```python
from build123d import *

# Parameters (mm, degrees)
REVOLVE_THIN1_OUTLINE_R                   = 10
REVOLVE_THIN1_DEPTH                       = 165
REVOLVE_THIN1_START                       = 15
REVOLVE_THIN1_2_OUTLINE_R                 = 12.5
REVOLVE_THIN1_2_OUTLINE_R_2               = 10
REVOLVE_THIN1_2_DEPTH                     = 10
F_5_0MM_DOWEL_HOLE1_D                     = 5
F_5_0MM_DOWEL_HOLE1_DEPTH                 = 10
F_5_0MM_DOWEL_HOLE1_CSINK_D               = 5.05
F_5_0MM_DOWEL_HOLE1_CSINK_ANGLE           = 90
F_5_0MM_DOWEL_HOLE1_TIP                   = 1.502151548
F_5_0MM_DOWEL_HOLE1_ON_FACE_2_D           = 5
F_5_0MM_DOWEL_HOLE1_ON_FACE_2_DEPTH       = 10
F_5_0MM_DOWEL_HOLE1_ON_FACE_2_CSINK_D     = 5.05
F_5_0MM_DOWEL_HOLE1_ON_FACE_2_CSINK_ANGLE = 90
F_5_0MM_DOWEL_HOLE1_ON_FACE_2_TIP         = 1.502151548
CUT_EXTRUDE1_DEPTH                        = 3


# Read off the part's stored shape, not the designer's step: Revolve-Thin1
with BuildPart() as part:
    # Revolve-Thin1 outline → Revolve-Thin1 (new body)
    with BuildSketch(Plane.YZ):
        Circle(REVOLVE_THIN1_OUTLINE_R)
    extrude(amount=REVOLVE_THIN1_DEPTH)

    # Revolve-Thin1 2 outline → Revolve-Thin1 2 (add)
    with BuildSketch(Plane.YZ.offset(REVOLVE_THIN1_START)):
        Circle(REVOLVE_THIN1_2_OUTLINE_R)
        Circle(REVOLVE_THIN1_2_OUTLINE_R_2, mode=Mode.SUBTRACT)
    extrude(amount=REVOLVE_THIN1_2_DEPTH)

    # Ø5.0mm Dowel Hole1
    with Locations(Plane(origin=(0, 0, 0), x_dir=(0, -1, 0), z_dir=(-1, 0, 0))):
        with Locations((0, 0)):
            CounterSinkHole(F_5_0MM_DOWEL_HOLE1_D / 2, F_5_0MM_DOWEL_HOLE1_CSINK_D / 2, depth=F_5_0MM_DOWEL_HOLE1_DEPTH, counter_sink_angle=F_5_0MM_DOWEL_HOLE1_CSINK_ANGLE)
            with Locations((0, 0, -(F_5_0MM_DOWEL_HOLE1_DEPTH + F_5_0MM_DOWEL_HOLE1_TIP / 2))):  # 118° drill point
                Cone(0, F_5_0MM_DOWEL_HOLE1_D / 2, F_5_0MM_DOWEL_HOLE1_TIP, mode=Mode.SUBTRACT)

    # Ø5.0mm Dowel Hole1 on face 2
    with Locations(Plane(origin=(165, 0, 0), x_dir=(0, 0, 1), z_dir=(1, 0, 0))):
        with Locations((0, 0)):
            CounterSinkHole(F_5_0MM_DOWEL_HOLE1_ON_FACE_2_D / 2, F_5_0MM_DOWEL_HOLE1_ON_FACE_2_CSINK_D / 2, depth=F_5_0MM_DOWEL_HOLE1_ON_FACE_2_DEPTH, counter_sink_angle=F_5_0MM_DOWEL_HOLE1_ON_FACE_2_CSINK_ANGLE)
            with Locations((0, 0, -(F_5_0MM_DOWEL_HOLE1_ON_FACE_2_DEPTH + F_5_0MM_DOWEL_HOLE1_ON_FACE_2_TIP / 2))):  # 118° drill point
                Cone(0, F_5_0MM_DOWEL_HOLE1_ON_FACE_2_D / 2, F_5_0MM_DOWEL_HOLE1_ON_FACE_2_TIP, mode=Mode.SUBTRACT)

    # Sketch3 → Cut-Extrude1 (cut)
    with BuildSketch(Plane(origin=(0, 10, 0), x_dir=(1, 0, 0), z_dir=(0, 1, 0))):
        with BuildLine():
            Line((28, 3), (47, 3))
            ThreePointArc((47, 3), (50, 0), (47, -3))
            Line((47, -3), (28, -3))
            ThreePointArc((28, -3), (25, 0), (28, 3))
        make_face()
        with BuildLine():
            Line((165, -3), (128, -3))
            ThreePointArc((128, -3), (125, 0), (128, 3))
            Line((128, 3), (165, 3))
            ThreePointArc((165, 3), (168, 0), (165, -3))
        make_face()
    extrude(amount=-CUT_EXTRUDE1_DEPTH, mode=Mode.SUBTRACT)


solid = part.part
```
Could you check a few things on this model? Use its own coordinates, in mm. A direction names the side the tool comes from. Round coordinates to 2 decimals unless told otherwise and drop trailing zeros. Order: outer loops, then holes, each group sorted by start corner. A loop starts at its lowest first (then second) coordinate and runs counter-clockwise, first axis right, second up. Notation, with made-up numbers: M 48.5,59.5 L 106.5,59.5 A15 cw 106.5,77.5 Z; hole C -16.75,71.5 d9. An arc over 180 degrees is marked long. One line per question, with ' | ' between items. Start each with the question number.
(1) Please list where these lines run through material, in increasing order: line 1 along Z through (x, y) = (6, 0); line 2 along Y through (x, z) = (160, 0); line 3 along X through (y, z) = (11, -1).
(2) Suppose I cut it at B-B on z = 6.5. List the corners of the cut face in (x, y) for me.
(3) For faces 1 (the face through (15, -0.1, 10.2)), 2 (the face through (94.02, -2.17, -9.76)), 3 (the face through (125, 9, 0)), which set-ups out of +Z, -Z, +X, -X, +Y, -Y let a thin tool reach every point of the face, with its end or its side?
(4) Suppose I cut it at A-A on y = -7.5. List the corners of the cut face in (x, z) for me.
(5) Thinking about a two-plate mould opening in X: for faces 4 (the face through (38, 7, 0)), 5 (the face through (153.759, 0.424, -0.094)), 6 (the face through (19.93, 11.923, 3.755)), which applies, +X half, -X half, draft (parallel to the pull), parting line (faces both ways), or undercut?
(6) Suppose I cut it at C-C on x = 82.5. List the corners of the cut face in (y, z) for me, then the cut area to 3 significant figures.
(7) For P1, Ø1, axis at x = 75, z = 7.5, coming from the +Y side; P2, Ø6.5, axis at x = 144.5, z = -1, coming from the +Y side; P3, Ø4.5, axis at y = 0, z = 0, coming from the -X side, each with a flat end and sliding along its axis, tell me the tip position at first contact or that it passes through.
Geometry results:
1) line 1: -10 to -2.5, 2.5 to 10 | line 2: -10 to -2.5, 2.5 to 7 | line 3: 15 to 25
2) outline: M 0,-7.6 L 15,-7.6 L 15,-10.68 L 25,-10.68 L 25,-7.6 L 165,-7.6 L 165,7.6 L 25,7.6 L 25,10.68 L 15,10.68 L 15,7.6 L 0,7.6 Z
3) face 1: -X | face 2: +X | face 3: +X, +Y
4) outline: M 0,-6.61 L 15,-6.61 L 15,-10 L 25,-10 L 25,-6.61 L 165,-6.61 L 165,6.61 L 25,6.61 L 25,10 L 15,10 L 15,6.61 L 0,6.61 Z
5) face 4: undercut | face 5: +X half | face 6: draft
6) outline: C 0,0 d20 | area: 314 mm²
7) P1: y = 7.14 | P2: y = 9.54 | P3: x = 10.15
